Model file for the job. Use its own axes, mm. A direction names the side the tool comes from. Give positions to 0.01 mm unless a question says otherwise; leave off trailing zeros. Order: outer loops, then holes, each group sorted by start corner. A loop starts at its lowest first (then second) coordinate and runs counter-clockwise, first axis right, second up. Notation, with made-up numbers: M 38.25,-1.5 L 73.25,-1.5 A9 cw 73.25,4.5 Z; hole C -3.75,89 d6. An arc over 180 degrees is marked long. Return JSON: item names as keys, results as strings. Group by question number.
1. Slice it at D-D on y = -12.5. List the corners of the cut face in (x, z) (1 decimal), then the cut area to 3 significant figures.
2. Slice it at A-A on z = 0. List the corners of the cut face in (x, y).
3. Slice it at B-B on x = 0. List the corners of the cut face in (y, z), then the cut area to 3 significant figures.
4. 3-axis set-ups, long thin cutter, end or side, ignore diameter. For faces 1 (the face through (5, -10, -5)), 2 (the face through (2.926, -2.535, 0.65)): which of +Z, -Z, +X, -X, +Y, -Y reach the whole face in a straight line?
5. Pin check, flat tips, straight feed: pin 1 (12 mm diameter, centred on x = 8, y = -10, fed in from -Z); pin 2 (2 mm diameter, centred on x = 5.5, y = -12, fed in from +Z); pin 3 (2 mm diameter, centred on x = 19.5, y = -23, fed in from -Z); pin 4 (12 mm diameter, centred on x = -9, z = -2, fed in from +Y). Stop position of each tip, or through.
6. Wall check: probe 1 along Y at (x, z) = (8.5, 5.5); probe 2 along Z at (x, y) = (0, -1.7); probe 3 along X at (y, z) = (-62.5, 12). Give the ranges that are in metal, low to high. Write a range as [from, to].
7. Slice it at C-C on y = -50. List the corners of the cut face in (x, z), then the cut area to 3 significant figures.
8. Two-plate mould, pull along Z, no slides. Class faces 3 (the face through (29.355, -40.56, 6.519)), 4 (the face through (5, 0, 0)), 5 (the face through (2.8, -5.3, -1.5)): released by +Z, released by -Z, zero draft, split by the parting line, or undercut.
from build123d import *


with BuildPart() as part:
    # Croquis2 → Revolución1 (revolve)
    with BuildSketch(Plane(origin=(0, 0, 0), x_dir=(0, 0, -1), z_dir=(1, 0, 0))):
        Polygon((0, 0), (25, 0), (35, -80), (20, -80), (11.25, -10), (0, -10), align=None)
    revolve(axis=Axis((0, -10, 0), (0, 1, 0)))

    # Croquis5 → Cortar-Revolución1 (revolve, cut)
    with BuildSketch(Plane(origin=(0, 0, 0), x_dir=(0, 0, -1), z_dir=(1, 0, 0))):
        Polygon((0, -10), (0, 0), (2.997515389, 0), (2.997515389, -5), (6, -10), align=None)
    revolve(axis=Axis((0, -10, 0), (0, 1, 0)), mode=Mode.SUBTRACT)


solid = part.part
Result:
{
 "1": {"outline": "C 0,0 d53.1; hole C 0,0 d23.1", "area": "1,800 mm2"},
 "2": {"outline": "M -35,-80 L -20,-80 L -11.25,-10 L -6,-10 L -3,-5 L -3,0 L -25,0 Z; M 3,-5 L 6,-10 L 11.25,-10 L 20,-80 L 35,-80 L 25,0 L 3,0 Z"},
 "3": {"outline": "M -80,-35 L 0,-25 L 0,-3 L -5,-3 L -10,-6 L -10,-11.25 L -80,-20 Z; M -80,20 L -10,11.25 L -10,6 L -5,3 L 0,3 L 0,25 L -80,35 Z", "area": "2,540 mm2"},
 "4": {"face 1": "-Y", "face 2": "+Y, -Y"},
 "5": {"pin 1": "stops at z = -26.52", "pin 2": "stops at z = 26.16", "pin 3": "stops at z = -20.87", "pin 4": "stops at y = 0"},
 "6": {"probe 1": "y = [-10, 0]", "probe 2": "z = [-25.21, -3], [3, 25.21]", "probe 3": "x = [-30.54, -13.16], [13.16, 30.54]"},
 "7": {"outline": "C 0,0 d62.5; hole C 0,0 d32.5", "area": "2,240 mm2"},
 "8": {"face 3": "split by the parting line", "face 4": "zero draft", "face 5": "undercut"}
}
